Input: dimensioned drawing with shaded views. Units: mm. Origin: part minimum x, y, z. A direction names the side the tool comes from. Coordinates: 2 decimals unless noted, no trailing zeros. Order: outer loops, then holes, each group sorted by start corner. A loop starts at its lowest first (then second) coordinate and runs counter-clockwise, first axis right, second up. Notation, with made-up numbers: (27, -33) -> (37, -33) arc R32 cw to (37, 4) -> close; hole circle Ø3 at (-32, -22). An arc over 180 degrees is marked (long way). Write item = value, one per line. Start each with the question number.
Item 1: Section query C-C (z = 41). Output: boundary loops of the cut face in (x, y).
Item 2: Ray query, line 1 along Y through (x, z) = (23.3, 9); line 2 along Y through (x, z) = (16, 4). Return the intervals inside material, ascending. Write a range as [from, to].
Item 3: Section query B-B (x = 21.75). Count the separate pieces of the cut face and the enclosed holes in it, then the cut area to 3 significant figures.
Item 4: Section query D-D (x = 8.5). Output: boundary loops of the cut face in (y, z), then the cut area to 3 significant figures.
Item 5: Set-up query: the marked faces 1, 2, 3, 4 and 5. Return all of +Z, -Z, +X, -X, +Y, -Y with unobstructed straight access to the full face (end or side cutting, diameter ignored); none if empty.
Item 6: Contact query for flat-ended pins moving along their axis: pin 1 (1.7 mm diameter, centred on y = 4, z = 46, fed in from +X); pin 2 (1 mm diameter, centred on y = 6, z = 10.5, fed in from +X); pin 3 (2 mm diameter, centred on x = 10.5, z = 40.5, fed in from -Y); pin 4 (6 mm diameter, centred on x = 7.5, y = 27, fed in from +Z). Output: stop coordinate, or through.
Item 7: Section query A-A (y = 46). Output: boundary loops of the cut face in (x, z).
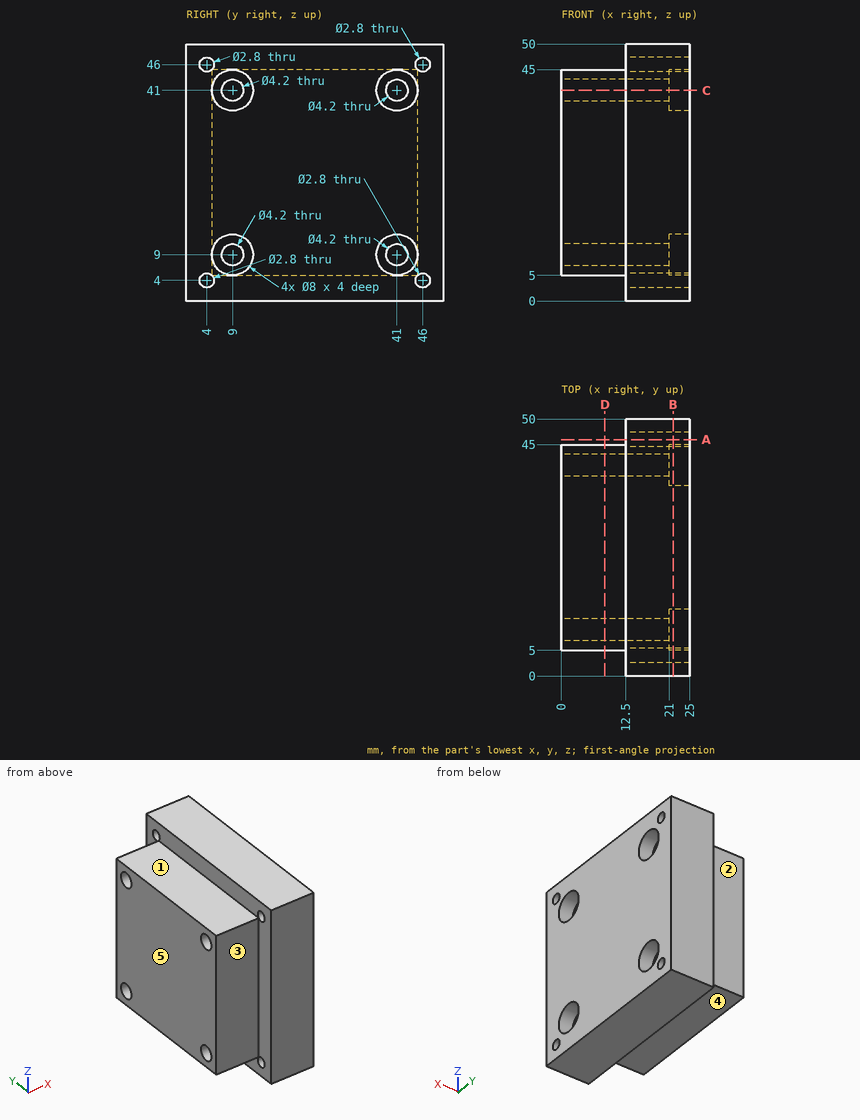
Computed:
q1.outline = (0, 5) -> (12.5, 5) -> (12.5, 0) -> (25, 0) -> (25, 5) -> (21, 5) -> (21, 6.9) -> (0, 6.9) -> close; (0, 11.1) -> (21, 11.1) -> (21, 13) -> (25, 13) -> (25, 37) -> (21, 37) -> (21, 38.9) -> (0, 38.9) -> close; (0, 43.1) -> (21, 43.1) -> (21, 45) -> (25, 45) -> (25, 50) -> (12.5, 50) -> (12.5, 45) -> (0, 45) -> close
q2.line_1 = [0, 5], [13, 37], [45, 50]
q2.line_2 = [0, 2.6], [5.4, 44.6], [47.4, 50]
q3.separate_pieces = 1
q3.enclosed_holes = 8
q3.area = 2,270 mm^2
q4.outline = (5, 5) -> (45, 5) -> (45, 45) -> (5, 45) -> close; hole circle Ø4.2 at (9, 9); hole circle Ø4.2 at (9, 41); hole circle Ø4.2 at (41, 9); hole circle Ø4.2 at (41, 41)
q4.area = 1,540 mm^2
q5.face_1 = +Z, -X, +Y, -Y
q5.face_2 = +Z, -Z, -X, +Y
q5.face_3 = +Z, -Z, -X, -Y
q5.face_4 = -Z, -X, +Y, -Y
q5.face_5 = +Z, -Z, -X, +Y, -Y
q6.pin_1 = through
q6.pin_2 = 21
q6.pin_3 = 5
q6.pin_4 = 45
q7.outline = (12.5, 0) -> (25, 0) -> (25, 2.6) -> (12.5, 2.6) -> close; (12.5, 5.4) -> (25, 5.4) -> (25, 44.6) -> (12.5, 44.6) -> close; (12.5, 47.4) -> (25, 47.4) -> (25, 50) -> (12.5, 50) -> close
